CAD build for the part. Positions are in the model's coordinates, mm. Round coordinates to 2 decimals unless told otherwise and drop trailing zeros. Loops run counter-clockwise (first coordinate to the right, second up) from the corner with the lowest first, then second, coordinate; pieces in that order, holes last. Notation, with made-up numbers: M -1.5,59.5 L 23.5,59.5 A18 ccw 23.5,86.5 Z; hole C 59.5,53 d6. An arc over 180 degrees is marked long. Put each result on its own line as item: value. Start each with the question number.
from build123d import *

# Parameters (mm, degrees)
SKETCH_1_W          = 295.949422796
SKETCH_1_H          = 458.479579913
EXTRUDE_1_DEPTH     = 64
SKETCH_2_W          = 64
SKETCH_2_H          = 308.479579913
CUT_EXTRUDE_1_DEPTH = 1028.33
SKETCH_3_W          = 63.9
SKETCH_3_H          = 149.8
CUT_EXTRUDE_2_DEPTH = 1028.33


with BuildPart() as part:
    # 스케치1 → 보스-돌출1 (new body)
    with BuildSketch(Plane.XY):
        with Locations((2908.978266494, -55.849619451)):
            Rectangle(SKETCH_1_W, SKETCH_1_H)
    extrude(amount=EXTRUDE_1_DEPTH)

    # 스케치2 → 컷-돌출1 (cut)
    with BuildSketch(Plane(origin=(3056.952977892, 0, 0), x_dir=(0, 0, -1), z_dir=(1, 0, 0))):
        with Locations((-32, 19.150380549)):
            Rectangle(SKETCH_2_W, SKETCH_2_H)
    extrude(amount=-CUT_EXTRUDE_1_DEPTH, mode=Mode.SUBTRACT)

    # 스케치3 → 컷-돌출2 (cut)
    with BuildSketch(Plane(origin=(3056.952977892, 0, 0), x_dir=(0, 0, -1), z_dir=(1, 0, 0))):
        with Locations((-31.95, -210.089409407)):
            Rectangle(SKETCH_3_W, SKETCH_3_H)
    extrude(amount=-CUT_EXTRUDE_2_DEPTH, mode=Mode.SUBTRACT)


solid = part.part
(1) Flat gauge pin, fed straight in: pin 1 Ø2 at (x, y) = (2860, -192.5) entering from -Z. Where does the tip first touch, or does it go through?
(2) Cut at A-A on z = 35.5. List the corners of the cut face in (x, y).
(3) Cut at B-B on x = 2956. List the corners of the cut face in (y, z), and give its area (3 significant figures).
(4) Cut at C-C on y = -196. List the corners of the cut face in (x, z).
Taken from the geometry:
1. pin 1: z = 63.9
2. outline: M 2761,-285.09 L 3056.95,-285.09 L 3056.95,-284.99 L 2761,-284.99 Z; M 2761,-135.19 L 3056.95,-135.19 L 3056.95,-135.09 L 2761,-135.09 Z
3. outline: M -285.09,0 L -284.99,0 L -284.99,63.9 L -135.19,63.9 L -135.19,0 L -135.09,0 L -135.09,64 L -285.09,64 Z
3. area: 27.8 mm2
4. outline: M 2761,63.9 L 3056.95,63.9 L 3056.95,64 L 2761,64 Z
